```python
from build123d import *

# Parameters (mm, degrees)
F1_DEPTH = 6
F0_W     = 228.6
F0_H     = 304.8
F2_DEPTH = 3


with BuildPart() as f1:
    # F0 (on Top) → F1 (new body)
    with BuildSketch(Plane.XY):
        with BuildLine():
            Line((19.558, 17.5422988832), (19.558, 19.5899201751))
            ThreePointArc((19.558, 19.5899201751), (19.4987310228, 18.0684562421), (19.3212833112, 16.5562136621))
            Line((19.3212833112, 16.5562136621), (19.558, 17.5422988832))
        make_face()
        with BuildLine():
            Line((1.5, 19.5899201751), (19.558, 19.5899201751))
            ThreePointArc((19.558, 19.5899201751), (-0.0281086289, 39.1478999763), (-19.5579192049, 19.5337029753))
            ThreePointArc((-19.5579192049, 19.5337029753), (-13.8097043416, 5.7404642292), (0, 0.0319201751))
            Line((0, 0.0319201751), (0, 18.0899201751))
            ThreePointArc((0, 18.0899201751), (-1.0606601718, 20.6505803469), (1.5, 19.5899201751))
        make_face()
        with BuildLine():
            ThreePointArc((0, 0.0319201751), (-13.8097043416, 5.7404642292), (-19.5579192049, 19.5337029753))
            Line((-19.5579192049, 19.5337029753), (-20.574, -20.0340798249))
            Line((-20.574, -20.0340798249), (10.5375261573, -20.0340798249))
            Line((10.5375261573, -20.0340798249), (18.5929127749, 13.5220574091))
            ThreePointArc((18.5929127749, 13.5220574091), (11.4856454765, 3.7597176499), (0, 0.0319201751))
        make_face()
        with BuildLine():
            ThreePointArc((-12.7889, -8.9850798249), (-15.3471702223, -10.0447500472), (-14.2875, -7.4864798249))
            ThreePointArc((-14.2875, -7.4864798249), (-13.2278297777, -7.9254096026), (-12.7889, -8.9850798249))
        make_face(mode=Mode.SUBTRACT)
        with BuildLine():
            ThreePointArc((1.5, -8.9850798249), (-1.0606601718, -10.0457399967), (0, -7.4850798249))
            ThreePointArc((0, -7.4850798249), (1.0606601718, -7.9244196531), (1.5, -8.9850798249))
        make_face(mode=Mode.SUBTRACT)
        with BuildLine():
            ThreePointArc((19.3212833112, 16.5562136621), (19.4987310228, 18.0684562421), (19.558, 19.5899201751))
            Line((19.558, 19.5899201751), (1.5, 19.5899201751))
            ThreePointArc((1.5, 19.5899201751), (1.0606601718, 18.5292600033), (0, 18.0899201751))
            Line((0, 18.0899201751), (0, 0.0319201751))
            ThreePointArc((0, 0.0319201751), (11.4856454765, 3.7597176499), (18.5929127749, 13.5220574091))
            Line((18.5929127749, 13.5220574091), (19.3212833112, 16.5562136621))
        make_face()
    extrude(amount=F1_DEPTH)

    # F0 (on Top) → F2 (join)
    with BuildSketch(Plane.XY):
        with Locations((33.862138617, 77.8095703363)):
            Rectangle(F0_W, F0_H)
        with BuildLine():
            ThreePointArc((-19.5579192049, 19.5337029753), (-0.0281086289, 39.1478999763), (19.558, 19.5899201751))
            Line((19.558, 19.5899201751), (19.558, 17.5422988832))
            Line((19.558, 17.5422988832), (19.558, -20.0340798249))
            Line((19.558, -20.0340798249), (10.5375261573, -20.0340798249))
            Line((10.5375261573, -20.0340798249), (-20.574, -20.0340798249))
            Line((-20.574, -20.0340798249), (-19.5579192049, 19.5337029753))
        make_face(mode=Mode.SUBTRACT)
    extrude(amount=F2_DEPTH)


solid = f1.part
```
Read the model definition and answer for the solid it produces. Units are mm, in the model's axes. Give positions to 0.01 mm unless a question says otherwise; leave off trailing zeros. Order: outer loops, then holes, each group sorted by start corner. A loop starts at its lowest first (then second) coordinate and runs counter-clockwise, first axis right, second up.
(1) Find section B-B (x = 87). Give the vertices of the cut face in (y, z).
(2) Find section C-C (y = 47.5). Give the vertices of the cut face in (x, z), plus the area to 3 significant figures.
(3) Find section A-A (z = 4.25). Give the vertices of the cut face in (x, y), plus the area to 3 significant figures.
(4) Straight lines are drawn through the part: L1, parallel to Z at x = -41.5, y = -56; L2, parallel to X at y = -4.5, z = 5.2; L3, parallel to X at y = 11, z = 4.9. For each, find the intervals that lie inside material, in ascending order.
(5) Given pin 1 (0.6 mm diameter, centred on y = 18.5, z = 5, fed in from +X); pin 2 (2.5 mm diameter, centred on x = -5.5, z = 5, fed in from -Y); pin 3 (5 mm diameter, centred on x = 0, y = 106.5, fed in from +Z), each flat-ended and moving along its own axis, determine where each tip first touches the part or whether it passes through.
Result sheet:
1. outline: (-74.59, 0) - (230.21, 0) - (230.21, 3) - (-74.59, 3) - close
2. outline: (-80.44, 0) - (148.16, 0) - (148.16, 3) - (-80.44, 3) - close
2. area: 686 mm2
3. outline: (-20.57, -20.03) - (10.54, -20.03) - (19.56, 17.54) - (19.56, 19.59) arc R19.56 ccw to (-19.56, 19.53) - close; hole circle Ø3 at (-14.29, -8.99); hole circle Ø3 at (0, -8.99); hole circle Ø3 at (0, 19.59)
3. area: 1,980 mm2
4. L1: z = 0 to 3
4. L2: x = -20.18 to 14.27
4. L3: x = -19.78 to 17.99
5. pin 1: stops at x = 19.56
5. pin 2: stops at y = -20.03
5. pin 3: stops at z = 3
